Autodesk Inventor part; units mm, degrees
ref_plane "YZ Plane" through (0, 0, 0) normal (1, 0, 0) x (0, 1, 0)
ref_plane "XZ Plane" through (0, 0, 0) normal (0, 1, 0) x (-1, 0, 0)
ref_plane "XY Plane" through (0, 0, 0) normal (0, 0, 1) x (1, 0, 0)
sketch "Sketch2" plane through (0, 0, 0) normal (0, 1, 0) x (-1, 0, 0)
  line L0 (-5.7, 5) -> (5.7, 5)
  line L1 (5.7, 5) -> (5.7, -5)
  line L2 (5.7, -5) -> (-5.7, -5)
  line L3 (-5.7, -5) -> (-5.7, 5)
  line L4 (-5.7, 5) -> (5.7, -5) construction
  line L5 (5.7, 5) -> (-5.7, -5) construction
  circle A0 centre (0, 0) radius 2.6
  dimension "d0" = 11.4
  dimension "d1" = 10
  dimension "d2" = 5.2
extrude "Extrusion1" add sketch "Sketch2" along normal blind 9
sketch "Sketch3" plane through (5.7, 0, -5) normal (0, 0, -1) x (-1, 0, 0)
  line L0 (0, 9) -> (11.4, 9)
  line L1 (0, 9) -> (0, 7)
  line L2 (0, 0) -> (0, 9)
  line L3 (0, 0) -> (0, 2)
  line L4 (0, 7) -> (0, 2)
  line L5 (0, 2) -> (11.4, 2)
  line L6 (11.4, 2) -> (11.4, 7)
  line L7 (11.4, 7) -> (0, 7)
  point P0 (5.7, 0)
  dimension "d5" = 2
  dimension "d6" = 2
extrude "Extrusion2" cut sketch "Sketch3" against normal blind 10.5875
sketch "Sketch4" plane through (0, 0, 0) normal (0, -1, 0) x (1, 0, 0)
  line L0 (-5.7, -5) -> (-5.7, 5)
  line L1 (-5.7, 5) -> (-5.7, 7)
  line L2 (-5.7, 7) -> (5.7, 7)
  line L3 (5.7, 7) -> (5.7, -7)
  line L4 (5.7, -7) -> (-5.7, -7)
  line L5 (-5.7, -7) -> (-5.7, 7)
  line L6 (-5.7, 7) -> (-5.7, -7)
  line L7 (-5.7, -7) -> (-7.7, -7)
  line L8 (-7.7, -7) -> (-7.7, 7)
  line L9 (-7.7, 7) -> (-5.7, 7)
  line L10 (5.7, -7) -> (5.7, -5)
  line L11 (5.7, -5) -> (-5.7, -5)
  line L12 (-5.7, -5) -> (-5.7, -7)
  line L13 (-5.7, -7) -> (5.7, -7)
  line L14 (-5.7, 5) -> (-5.7, 7)
  line L15 (-5.7, 7) -> (5.7, 7)
  line L16 (5.7, 7) -> (5.7, 5)
  line L17 (5.7, 5) -> (-5.7, 5)
  line L18 (-5.7, -5) -> (-5.7, 5)
  line L19 (5.7, -5) -> (5.7, 5)
  point P0 (0, 0)
  dimension "d9" = 2
  dimension "d10" = 11.4
  dimension "d11" = 14
  dimension "d12" = 2
extrude "Extrusion3" add sketch "Sketch4" against normal up to surface (9 mm away) contours L11 L3 L4 L5 | L1 L2 L3 L17
sketch "Sketch6" plane through (0, 9, 0) normal (0, 1, 0) x (1, 0, 0)
  circle A0 centre (0, 0) radius 3.1
  dimension "d18" = 6.2
extrude "Extrusion4" cut sketch "Sketch6" against normal blind 10
Source: CAD feature listing. Evaluate the final solid. Frame: model axes, mm. A direction names the side the tool comes from. Give positions to 0.01 mm unless a question says otherwise; leave off trailing zeros. Loops run counter-clockwise (first coordinate to the right, second up) from the corner with the lowest first, then second, coordinate; pieces in that order, holes last. Notation, with made-up numbers: (-32, -30) - (27, -30) arc R23 ccw to (27, -17) - close; hole circle Ø2 at (20, -29). An arc over 180 degrees is marked (long way). Use CSV: the item, a comma, the result in double quotes. Start each with the question number.
1. Ray query, L1, parallel to Y at x = -4.25, z = -3.75; L2, parallel to Z at x = 0, y = 0.6; L3, parallel to X at y = 7.4, z = 0. Return the intervals inside material, ascending.
2. Section B-B (z = 0). Output: boundary loops of the cut face in (x, y), then the cut area to 3 significant figures.
3. Section C-C (y = 1.25). Output: boundary loops of the cut face in (x, z).
4. Section A-A (x = 0). Output: boundary loops of the cut face in (y, z), then the cut area to 3 significant figures.
5. Section D-D (y = 2.25). Output: boundary loops of the cut face in (x, z), then the cut area to 3 significant figures.
6. Reachability of faces 1 (the flat face through (0, 4, -7)), 2 (the flat face through (0.1, 2, -3.4)) from +Z, -Z, +X, -X, +Y, -Y: full face, straight path, thin tool, end or side. Return the list, or none.
7. Pin query (flat end, axial travel): pin 1 (3.5 mm diameter, centred on x = 0, z = 0, fed in from -Y). Return the tip coordinate at first contact, or that it passes through.
8. Draft query along Y for faces 3 (the flat face through (0, 4, 5)), 4 (the flat face through (1.3, 0, 3.2)), 5 (the flat face through (0, 4, 7)). Return one class per face: +Y half, -Y half, draft (parallel to the pull), parting line (faces both ways), or undercut.
Response:
1,L1,"0 to 2, 7 to 9"
1,L2,"-7 to -3.1, 3.1 to 7"
1,L3,"-5.7 to -3.1, 3.1 to 5.7"
2,outline,"(-5.7, 0) - (-3.1, 0) - (-3.1, 2) - (-5.7, 2) - close; (-5.7, 7) - (-3.1, 7) - (-3.1, 9) - (-5.7, 9) - close; (3.1, 0) - (5.7, 0) - (5.7, 2) - (3.1, 2) - close; (3.1, 7) - (5.7, 7) - (5.7, 9) - (3.1, 9) - close"
2,area,"20.8 mm²"
3,outline,"(-5.7, -7) - (5.7, -7) - (5.7, 7) - (-5.7, 7) - close; hole circle Ø6.2 at (0, 0)"
4,outline,"(0, -7) - (9, -7) - (9, -3.1) - (7, -3.1) - (7, -5) - (2, -5) - (2, -3.1) - (0, -3.1) - close; (0, 3.1) - (2, 3.1) - (2, 5) - (7, 5) - (7, 3.1) - (9, 3.1) - (9, 7) - (0, 7) - close"
4,area,"51.2 mm²"
5,outline,"(-5.7, -7) - (5.7, -7) - (5.7, -5) - (-5.7, -5) - close; (-5.7, 5) - (5.7, 5) - (5.7, 7) - (-5.7, 7) - close"
5,area,"45.6 mm²"
6,face 1,"-Z, +X, -X, +Y, -Y"
6,face 2,"+X, -X"
7,pin 1,"through"
8,face 3,"undercut"
8,face 4,"-Y half"
8,face 5,"draft"
